from build123d import *

# Parameters (mm, degrees)
BOSS_EXTRUDE1_DEPTH = 7
BOSS_EXTRUDE2_DEPTH = 5
CHAMFER1_SIZE       = 12.5
CHAMFER1_SIZE2      = 4.549627928


with BuildPart() as part:
    # Sketch1 → Boss-Extrude1 (new body)
    with BuildSketch(Plane(origin=(0, 0, 0), x_dir=(1, 0, 0), z_dir=(0, 1, 0))):
        with BuildLine():
            Line((-32.5, 55), (-32.5, -55))
            ThreePointArc((-32.5, -55), (0, -60.156372261), (32.5, -55))
            Line((32.5, -55), (32.5, 55))
            ThreePointArc((32.5, 55), (0, 60.156372261), (-32.5, 55))
        make_face()
    extrude(amount=BOSS_EXTRUDE1_DEPTH)

    # Sketch2 → Boss-Extrude2 (add)
    with BuildSketch(Plane(origin=(0, 7, 0), x_dir=(1, 0, 0), z_dir=(0, 1, 0))):
        with BuildLine():
            Line((29.9, -53.093852319), (29.9, 53.093852319))
            ThreePointArc((29.9, 53.093852319), (0, 57.556372261), (-29.9, 53.093852319))
            Line((-29.9, 53.093852319), (-29.9, -53.093852319))
            ThreePointArc((-29.9, -53.093852319), (0, -57.556372261), (29.9, -53.093852319))
        make_face()
        with BuildLine():
            Line((28.4, -51.977082856), (28.4, 51.977082856))
            ThreePointArc((28.4, 51.977082856), (0, 56.056372261), (-28.4, 51.977082856))
            Line((-28.4, 51.977082856), (-28.4, -51.977082856))
            ThreePointArc((-28.4, -51.977082856), (0, -56.056372261), (28.4, -51.977082856))
        make_face(mode=Mode.SUBTRACT)
    extrude(amount=BOSS_EXTRUDE2_DEPTH)

    # Chamfer1
    chamfer1_edges = [part.edges().sort_by_distance(p)[0] for p in [
        (-32.5, 0, 0),
        (0, 0, -60.156372261),
        (32.5, 0, 0),
        (0, 0, 60.156372261),
    ]]
    chamfer1_side = [part.faces().sort_by_distance(p)[0] for p in [
        (0, 0, 0),
    ]]
    chamfer(chamfer1_edges, length=CHAMFER1_SIZE, length2=CHAMFER1_SIZE2, reference=chamfer1_side[0])


solid = part.part
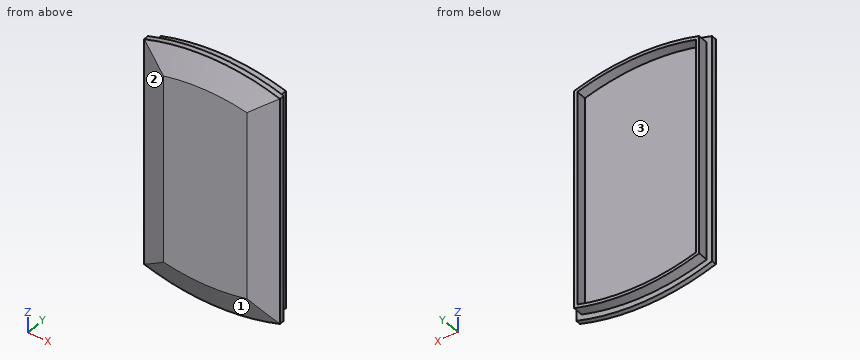
CAD build for the part. Positions are in the model's coordinates, mm. Face numbers are marked on the shaded views. Round coordinates to 2 decimals unless told otherwise and drop trailing zeros. Loops run counter-clockwise (first coordinate to the right, second up) from the corner with the lowest first, then second, coordinate; pieces in that order, holes last. Notation, with made-up numbers: (-19, 71) - (-4, 71) arc R16 cw to (-4, 81) - close; hole circle Ø10 at (36.5, -32). An arc over 180 degrees is marked (long way). Put each result on its own line as item: value.
1. Slice it at B-B on z = -16.5. List the corners of the cut face in (x, y).
Geometry check:
outline: (-32.5, 4.55) - (-20, 0) - (20, 0) - (32.5, 4.55) - (32.5, 7) - (29.9, 7) - (29.9, 12) - (28.4, 12) - (28.4, 7) - (-28.4, 7) - (-28.4, 12) - (-29.9, 12) - (-29.9, 7) - (-32.5, 7) - close
2. Slice it at A-A on y = 10.5. List the corners of the cut face in (x, z).
Geometry check:
outline: (-29.9, -53.09) arc R102.4 ccw to (29.9, -53.09) - (29.9, 53.09) arc R102.4 ccw to (-29.9, 53.09) - close; hole (-28.4, -51.98) arc R100.9 ccw to (28.4, -51.98) - (28.4, 51.98) arc R100.9 ccw to (-28.4, 51.98) - close
3. Slice it at C-C on y = 1.25. List the corners of the cut face in (x, z), and give its area (3 significant figures).
Geometry check:
outline: (-23.43, -48.18) arc R95.93 ccw to (23.43, -48.18) - (23.43, 48.18) arc R95.93 ccw to (-23.43, 48.18) - close
area: 4,700 mm²
4. Wall check: line 1 (X direction, y = 11.25, z = -12); line 2 (Z direction, x = -0.5, y = 9.25); line 3 (Z direction, x = 22, y = 8). Give the ranges that are in metal, low to high.
Geometry check:
line 1: -29.9 to -28.4, 28.4 to 29.9
line 2: -57.56 to -56.06, 56.06 to 57.56
line 3: -55.17 to -53.63, 53.63 to 55.17
5. Pin check, flat tips, straight feed: P1, Ø3, axis at x = 22, z = 22.5, coming from the +Y side; P2, Ø5.5, axis at y = 10.5, z = 21.5, coming from the -X side; P3, Ø1.5, axis at y = 8.5, z = -14.5, coming from the +X side. Stop position of each tip, or through.
Geometry check:
P1: y = 7
P2: x = -29.9
P3: x = 29.9
6. Two-plate mould, pull along Z, no slides. Class the marked faces 1, 2 and 3: released by +Z, released by -Z, zero draft, split by the parting line, or undercut.
Geometry check:
face 1: released by -Z
face 2: zero draft
face 3: undercut
